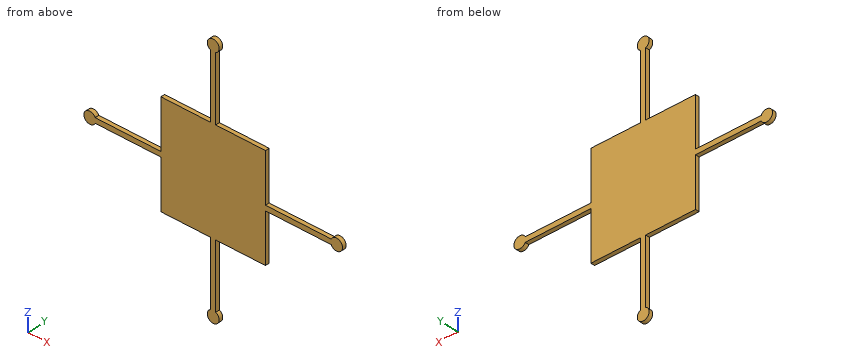
```python
from build123d import *

# Parameters (mm, degrees)
BOSS_EXTRUDE1_DEPTH = 2.54


with BuildPart() as part:
    # Sketch1 → Boss-Extrude1 (new body)
    with BuildSketch(Plane(origin=(0, 0, 0), x_dir=(1, 0, 0), z_dir=(0, 1, 0))):
        with BuildLine():
            Line((34.356030095, 0), (65.506126721, 0))
            Line((65.506126721, 0), (65.506126721, 31.150096626))
            Line((65.506126721, 31.150096626), (106.681389714, 31.150096626))
            ThreePointArc((106.681389714, 31.150096626), (113.737222592, 32.753063361), (106.681389714, 34.356030095))
            Line((106.681389714, 34.356030095), (65.506126721, 34.356030095))
            Line((65.506126721, 34.356030095), (65.506126721, 65.506126721))
            Line((65.506126721, 65.506126721), (34.356030095, 65.506126721))
            Line((34.356030095, 65.506126721), (34.356030095, 106.681389714))
            ThreePointArc((34.356030095, 106.681389714), (32.753063361, 113.737222592), (31.150096626, 106.681389714))
            Line((31.150096626, 106.681389714), (31.150096626, 65.506126721))
            Line((31.150096626, 65.506126721), (0, 65.506126721))
            Line((0, 65.506126721), (0, 34.356030095))
            Line((0, 34.356030095), (-41.175262993, 34.356030095))
            ThreePointArc((-41.175262993, 34.356030095), (-48.231095871, 32.753063361), (-41.175262993, 31.150096626))
            Line((-41.175262993, 31.150096626), (0, 31.150096626))
            Line((0, 31.150096626), (0, 0))
            Line((0, 0), (31.150096626, 0))
            Line((31.150096626, 0), (31.150096626, -41.175262993))
            ThreePointArc((31.150096626, -41.175262993), (32.753063361, -48.231095871), (34.356030095, -41.175262993))
            Line((34.356030095, -41.175262993), (34.356030095, 0))
        make_face()
    extrude(amount=BOSS_EXTRUDE1_DEPTH)


solid = part.part
```
The model under review builds one solid part; all positions refer to its coordinate system, in mm. Round coordinates to 2 decimals unless told otherwise and drop trailing zeros. Write each loop counter-clockwise with the first axis right and the second up, starting at its lowest first coordinate (ties: lowest second). Pieces come first, ordered by that corner, then holes.
(1) We need section B-B on z = 31.5. Give the boundary of the cut face in (x, y), and give its area (3 significant figures).
(2) Wall thickness on L1, parallel to Z at x = 83, y = 1.2; L2, parallel to Z at x = 26, y = 1.75; L3, parallel to X at y = 2.25, z = -35: over which ranges is each line inside the solid? List them lowest first.
(3) We need section A-A on y = 1.55. Give the boundary of the cut face in (x, z), and give its area (3 significant figures).
(4) Insertion check: pin 1 (0.8 mm diameter, centred on y = 1, z = 26, fed in from +X); pin 2 (1.3 mm diameter, centred on y = 1, z = -43.5, fed in from +X); pin 3 (1.3 mm diameter, centred on x = 12.5, y = 1.5, fed in from +Z). Each pin has a flat end and moves straight along its axis. Give the tip position at first contact, or say it passes through.
(5) We need section C-C on x = -26. Give the boundary of the cut face in (y, z).
Findings below:
1. outline: (31.15, 0) - (34.36, 0) - (34.36, 2.54) - (31.15, 2.54) - close
1. area: 8.14 mm2
2. L1: z = -34.36 to -31.15
2. L2: z = -65.51 to 0
2. L3: x = -47.47 to -41.57, 0 to 65.51, 107.08 to 112.98
3. outline: (-41.18, -34.36) - (0, -34.36) - (0, -65.51) - (31.15, -65.51) - (31.15, -106.68) arc R3.71 ccw (long way) to (34.36, -106.68) - (34.36, -65.51) - (65.51, -65.51) - (65.51, -34.36) - (106.68, -34.36) arc R3.71 ccw (long way) to (106.68, -31.15) - (65.51, -31.15) - (65.51, 0) - (34.36, 0) - (34.36, 41.18) arc R3.71 ccw (long way) to (31.15, 41.18) - (31.15, 0) - (0, 0) - (0, -31.15) - (-41.18, -31.15) arc R3.71 ccw (long way) to start
3. area: 4,990 mm2
4. pin 1: stops at x = 34.36
4. pin 2: stops at x = 65.51
4. pin 3: stops at z = 0
5. outline: (0, -34.36) - (2.54, -34.36) - (2.54, -31.15) - (0, -31.15) - close
